from build123d import *

# Parameters (mm, degrees)
SKETCH1_R           = 1.75
BOSS_EXTRUDE1_DEPTH = 8.5
CUT_EXTRUDE2_DEPTH  = 2.5
CUT_EXTRUDE3_DEPTH  = 2.5
SKETCH5_R           = 3.5
CUT_EXTRUDE4_DEPTH  = 3.5
SKETCH6_R           = 3.5
CUT_EXTRUDE5_DEPTH  = 3.5
FILLET1_R           = 11.4
SKETCH7_W           = 8.501662988
SKETCH7_H           = 41.75
BOSS_EXTRUDE3_DEPTH = 8.5
FILLET2_R           = 5
FILLET3_R           = 5


with BuildPart() as part:
    # Sketch1 → Boss-Extrude1 (new body)
    with BuildSketch(Plane.XY):
        Polygon((8, -10), (8, -27), (-25, -27), (-25, 14.75), align=None)
        with Locations((-20, 1)):
            Circle(SKETCH1_R, mode=Mode.SUBTRACT)
        with Locations((0, -14)):
            Circle(SKETCH1_R, mode=Mode.SUBTRACT)
        Polygon((-6.687894354, -19), (-6.666666667, -19), (-6.687894354, -18.984079234), align=None, mode=Mode.SUBTRACT)
    extrude(amount=BOSS_EXTRUDE1_DEPTH)

    # Sketch3 → Cut-Extrude2 (cut)
    with BuildSketch(Plane(origin=(0, 0, 0), x_dir=(-1, 0, 0), z_dir=(0, 0, -1))):
        Polygon((22.725, 2.573279484), (20, 4.146558967), (17.275, 2.573279484), (17.275, -0.573279484), (20, -2.146558967), (22.725, -0.573279484), align=None)
    extrude(amount=-CUT_EXTRUDE2_DEPTH, mode=Mode.SUBTRACT)

    # Sketch4 → Cut-Extrude3 (cut)
    with BuildSketch(Plane.XY.offset(8.5)):
        Polygon((-2.517247174, -12.11206462), (-2.893623587, -15.23603231), (-0.376376413, -17.12396769), (2.517247174, -15.88793538), (2.893623587, -12.76396769), (0.376376413, -10.87603231), align=None)
    extrude(amount=-CUT_EXTRUDE3_DEPTH, mode=Mode.SUBTRACT)

    # Sketch5 → Cut-Extrude4 (cut)
    with BuildSketch(Plane.XY.offset(8.5)):
        with Locations((-20, 1)):
            Circle(SKETCH5_R)
    extrude(amount=-CUT_EXTRUDE4_DEPTH, mode=Mode.SUBTRACT)

    # Sketch6 → Cut-Extrude5 (cut)
    with BuildSketch(Plane(origin=(0, 0, 0), x_dir=(-1, 0, 0), z_dir=(0, 0, -1))):
        with Locations((0, -14)):
            Circle(SKETCH6_R)
    extrude(amount=-CUT_EXTRUDE5_DEPTH, mode=Mode.SUBTRACT)

    # Fillet1
    # the kernel refuses this fillet: 11.4 mm, written as the material it takes off along each edge
    with BuildSketch(Plane(origin=(8, -10, -14.25), x_dir=(0, -1, 0), z_dir=(0, 0, 1))) as fillet1_piece_1:
        with BuildLine():
            CenterArc((FILLET1_R * 0.5, -FILLET1_R), FILLET1_R, 90, 53.130102354)
            Line((-FILLET1_R * 0.3, -FILLET1_R * 0.4), (0, 0))
            Line((0, 0), (FILLET1_R * 0.5, 0))
        make_face()
    extrude(amount=37, mode=Mode.SUBTRACT)
    with BuildSketch(Plane(origin=(8, -27, -28.5), x_dir=(0, 1, 0), z_dir=(0, 0, 1))) as fillet1_piece_2:
        with BuildLine():
            CenterArc((FILLET1_R, FILLET1_R), FILLET1_R, 180, 90)
            Line((0, FILLET1_R), (0, 0))
            Line((0, 0), (FILLET1_R, 0))
        make_face()
    extrude(amount=65.5, mode=Mode.SUBTRACT)

    # Sketch7 → Boss-Extrude3 (add)
    with BuildSketch(Plane.ZY.offset(25)):
        with Locations((4.25, -6.125)):
            Rectangle(SKETCH7_W, SKETCH7_H)
    extrude(amount=BOSS_EXTRUDE3_DEPTH)

    # Fillet2
    fillet2_edges = [part.edges().sort_by_distance(p)[0] for p in [
        (-33.5, -27, 4.25),
    ]]
    fillet(fillet2_edges, radius=FILLET2_R)

    # Fillet3
    fillet3_edges = [part.edges().sort_by_distance(p)[0] for p in [
        (-33.5, 14.75, 4.25),
    ]]
    fillet(fillet3_edges, radius=FILLET3_R)


solid = part.part
Source: CAD feature listing. Evaluate the final solid. Frame: model axes, mm. A direction names the side the tool comes from. Give positions to 0.01 mm unless a question says otherwise; leave off trailing zeros. Write each loop counter-clockwise with the first axis right and the second up, starting at its lowest first coordinate (ties: lowest second). Pieces come first, ordered by that corner, then holes. Notation, with made-up numbers: (33, 56.5) -> (41, 56.5) arc R17 cw to (41, 85.5) -> close; hole circle Ø7 at (-31, -24). An arc over 180 degrees is marked (long way). Return JSON: item names as keys, results as strings. Group by question number.
1. Section C-C, the plane x = -15. Output: boundary loops of the cut face in (y, z), then the cut area to 3 significant figures.
2. Pin query (flat end, axial travel): pin 1 Ø7.5 at (x, y) = (-21, 2) entering from +Z; pin 2 Ø2 at (x, y) = (0, -14) entering from -Z; pin 3 Ø4 at (x, y) = (0, -14) entering from +Z; pin 4 Ø1 at (y, z) = (-12, 1) entering from +X. Return the tip coordinate at first contact, or that it passes through.
3. Access query for faces 4 (the face through (-18.62, -1.35, 1.23)), 5 (the face through (2, -14, 6)), 6 (the face through (6.82, -10.65, 4.19)). Directions: +Z, -Z, +X, -X, +Y, -Y. A direction counts if a zero-diameter tool reaches every point of the face in a straight line with its end or side. Return the directions, or none.
4. Material intervals for line 1 (Y direction, x = 0, z = 2.8); line 2 (X direction, y = 3, z = 5.5); line 3 (X direction, y = -16.5, z = 7), sorted ascending. Write a range as from..to.
5. Mould query, pull axis Y, two halves, no side actions, for faces 1 (the face through (-32, -25.57, 4.31)), 2 (the face through (-29, -6, 8.501)), 3 (the face through (1.65, -11.83, 7.27)). Classes: +Y half, -Y half, draft (parallel to the pull), parting line (faces both ways), or undercut.
Determined:
{
 "1": {"outline": "(-27, 0) -> (7.25, 0) -> (7.25, 8.5) -> (-27, 8.5) -> close", "area": "291 mm2"},
 "2": {"pin 1": "stops at z = 8.5", "pin 2": "passes through", "pin 3": "stops at z = 6", "pin 4": "stops at x = 7.54"},
 "3": {"face 4": "-Z", "face 5": "+Z", "face 6": "+Z, -Z, +X, +Y"},
 "4": {"line 1": "y = -26.48..-17.5, -10.5..-4", "line 2": "x = -33.5..-22.87, -17.13..-9.33", "line 3": "x = -33.5..-1.21, 1.08..7.96"},
 "5": {"face 1": "-Y half", "face 2": "draft", "face 3": "undercut"}
}
